Part model, mm, in its own coordinate system. A direction names the side the tool comes from. Coordinates: 2 decimals unless noted, no trailing zeros. Write each loop counter-clockwise with the first axis right and the second up, starting at its lowest first coordinate (ties: lowest second). Pieces come first, ordered by that corner, then holes. Notation, with made-up numbers: M 62,71 L 72,71 A19 cw 72,76 Z; hole C 71.5,-3 d4. An arc over 180 degrees is marked long. Use a Markdown table: item, result. Add a question column.
Q1. Tool access for faces 1 (the flat face through (105, 56.1, 17)), 2 (the flat face through (201.6, 30, 17)), 3 (the flat face through (103, 4.5, 17)): list every direction of +Z, -Z, +X, -X, +Y, -Y with a clear straight run to the whole face (end or side of a thin tool).
Q2. Slice it at A-A on x = 64. Write the cut outline in (y, z).
Q3. Pin check, flat tips, straight feed: pin 1 Ø10 at (y, z) = (14, 7.5) entering from -X; pin 2 Ø1 at (y, z) = (41, 17) entering from -X; pin 3 Ø1.9 at (x, y) = (198, 30.3) entering from -Z; pin 4 Ø1 at (x, z) = (135, 16.5) entering from -Y. Stop position of each tip, or through.
Q4. Wall check: L1, parallel to X at y = 30.3, z = 7.5; L2, parallel to Y at x = 198, z = 9.75; L3, parallel to Z at x = 114, y = 2. Give the ranges that are in metal, low to high. Write a range as from..to.
Autodesk Inventor part; units mm, degrees
ref_plane "YZ Plane" through (0, 0, 0) normal (1, 0, 0) x (0, 1, 0)
ref_plane "XZ Plane" through (0, 0, 0) normal (0, 1, 0) x (-1, 0, 0)
ref_plane "XY Plane" through (0, 0, 0) normal (0, 0, 1) x (1, 0, 0)
sketch "スケッチ1" plane through (0, 0, 0) normal (0, 0, 1) x (1, 0, 0)
  line L0 (0, 0) -> (208, 0)
  line L1 (208, 0) -> (208, 60.6)
  line L2 (208, 60.6) -> (0, 60.6)
  line L3 (0, 60.6) -> (0, 0)
  line L4 (6.4, 4.5) -> (201.6, 4.5)
  line L5 (201.6, 4.5) -> (201.6, 56.1)
  line L6 (201.6, 56.1) -> (6.4, 56.1)
  line L7 (6.4, 56.1) -> (6.4, 4.5)
  dimension "d0" = 208
  dimension "d1" = 60.6
  dimension "d2" = 195.2
  dimension "d3" = 51.6
extrude "押し出し1" add sketch "スケッチ1" along normal blind 15.2
extrude "押し出し2" add sketch "スケッチ1" along normal blind 18.5 contours L7 L6 L5 L4
sketch "スケッチ2" plane through (0, 0, 0) normal (0, 0, -1) x (-1, 0, 0)
  line L0 (0, 60.6) -> (0, 0)
  line L1 (-208, 0) -> (-208, 60.6)
  line L2 (0, 0) -> (-208, 0)
  point P0 (-198, 30.3)
  point P1 (-10, 30.3)
  dimension "d8" = 10
  dimension "d9" = 10
  dimension "d19" = 30.3
  dimension "d22" = 30.3
hole "穴1" at (198, 30.3, 0) at (10, 30.3, 0) direction (0, 0, 1) diameter 3.2 end through all
properties part number "TH22_soroban_sn" material "ABS プラスチック"
Recorded:
| question | item | result |
|---|---|---|
| 1 | face 1 | +Z, +X, -X, +Y |
| 1 | face 2 | +Z, +X, +Y, -Y |
| 1 | face 3 | +Z, +X, -X, -Y |
| 2 | outline | M 0,0 L 60.6,0 L 60.6,15.2 L 56.1,15.2 L 56.1,18.5 L 4.5,18.5 L 4.5,15.2 L 0,15.2 Z |
| 3 | pin 1 | x = 0 |
| 3 | pin 2 | x = 6.4 |
| 3 | pin 3 | through |
| 3 | pin 4 | y = 4.5 |
| 4 | L1 | 0..8.4, 11.6..196.4, 199.6..208 |
| 4 | L2 | 0..28.7, 31.9..60.6 |
| 4 | L3 | 0..15.2 |
